The figure shows three views and two pictorial views of one solid part (mm, origin at its lowest corner). Answer the questions. A direction names the side the tool comes from. Give positions to 0.01 mm unless a question says otherwise; leave off trailing zeros. Order: outer loops, then holes, each group sorted by start corner. A loop starts at its lowest first (then second) coordinate and runs counter-clockwise, first axis right, second up. Notation, with made-up numbers: (79.5, 51.25) - (105.5, 51.25) arc R33 cw to (105.5, 90.25) - close; hole circle Ø4 at (5, 41). An arc over 180 degrees is marked (long way). Return JSON: item names as keys, results as strings. Group by question number.
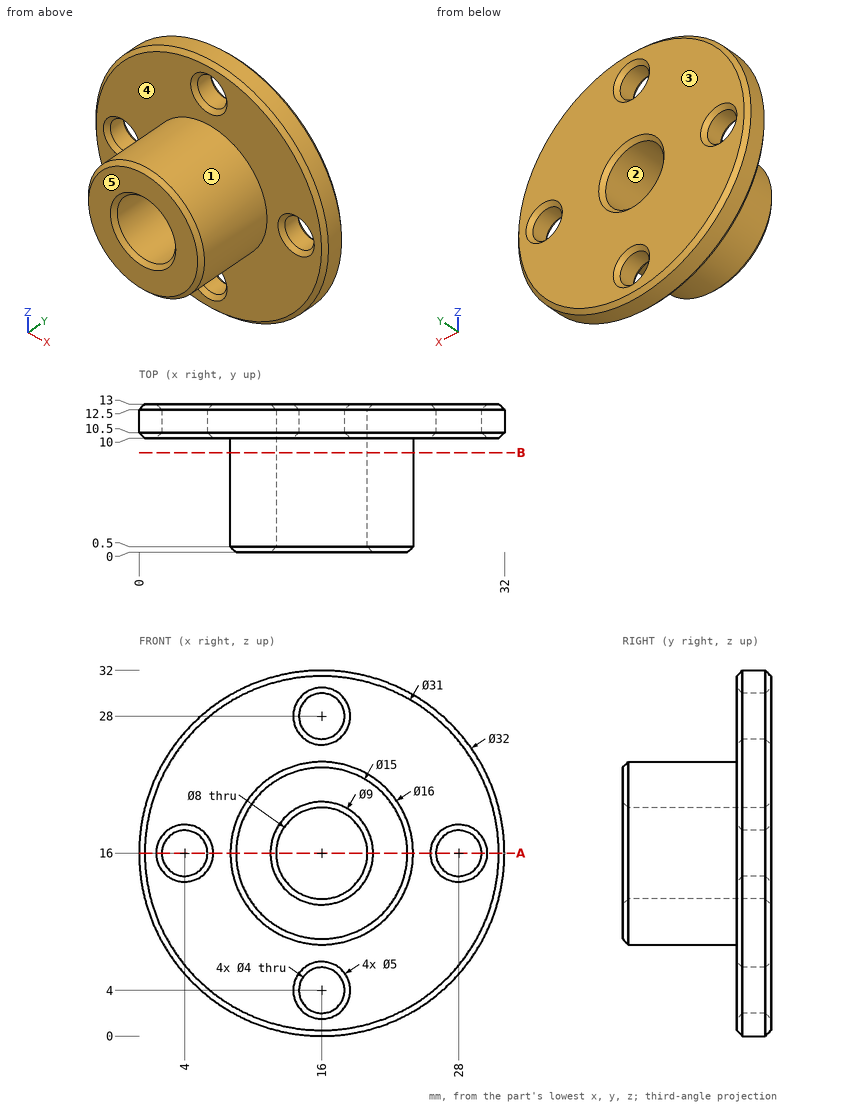
1. Determine the mould class of the marked faces 1, 2 and 3 for opening direction Z: released by +Z, released by -Z, zero draft, split by the parting line, or undercut.
2. Consider probe 1 along Z at (x, y) = (16, 12.15); probe 2 along Z at (x, y) = (16, 4.75); probe 3 along Y at (x, z) = (3.5, 20). Determine where each line is inside the solid, lowest interval first. Write a range as from..to.
3. Each of these flat-tipped pins is pushed along its axis until it touches: pin 1 (4.5 mm diameter, centred on x = 16, z = 28, fed in from +Y); pin 2 (4 mm diameter, centred on y = 10, z = 4, fed in from -X); pin 3 (8 mm diameter, centred on x = 12.5, z = 3, fed in from -Y); pin 4 (3.5 mm diameter, centred on x = 4, z = 16, fed in from +Y). Where does it stop, or does it pass through?
4. The part is cut by section A-A (z = 16). State how many separate pieces and enclosed holes the cut face has, and give its area (3 significant figures).
5. The part is cut by section B-B (y = 8.75). Give the vertices of the cut face in (x, z).
6. A tool of negligible diameter and unlimited length cuts with its end or side. For the marked faces 4 and 5, from which of +Z, -Z, +X, -X, +Y, -Y can it reach the whole face along a straight path? Write none if from no direction.
Answers:
{
 "1": {"face 1": "split by the parting line", "face 2": "undercut", "face 3": "zero draft"},
 "2": {"probe 1": "z = 0..2, 6..12, 20..26, 30..32", "probe 2": "z = 8..12, 20..24", "probe 3": "y = 10..13"},
 "3": {"pin 1": "stops at y = 12.75", "pin 2": "stops at x = 3.56", "pin 3": "stops at y = 10", "pin 4": "passes through"},
 "4": {"separate pieces": "4", "enclosed holes": "0", "area": "126 mm^2"},
 "5": {"outline": "circle Ø16 at (16, 16); hole circle Ø8 at (16, 16)"},
 "6": {"face 4": "-Y", "face 5": "+Z, -Z, +X, -X, -Y"}
}
